Check sheet for the drawn part. Datum: minimum x, y, z corner. Units: mm. Round coordinates to 2 decimals unless told otherwise and drop trailing zeros. Write each loop counter-clockwise with the first axis right and the second up, starting at its lowest first coordinate (ties: lowest second). Pieces come first, ordered by that corner, then holes. Notation, with made-up numbers: (41, -27.75) - (98, -27.75) arc R27 ccw to (98, 5.25) - close; hole circle Ø6 at (81, 11). An arc over 180 degrees is marked (long way). Answer as a JSON object with one key per item and string values.
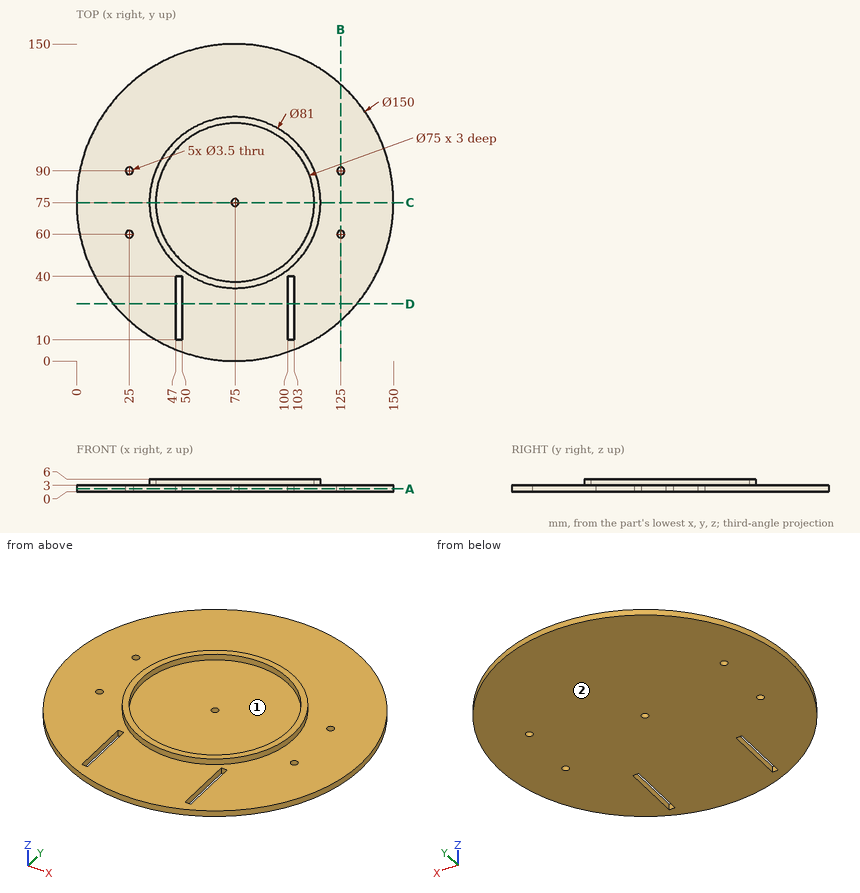
Q1. Section check A-A, the plane z = 1.35. Record the cut outline in (x, y), then the cut area to 3 significant figures.
Geometry check:
{"outline": "circle Ø150 at (75, 75); hole circle Ø3.5 at (25, 60); hole circle Ø3.5 at (25, 90); hole (47, 10) - (50, 10) - (50, 40) - (47, 40) - close; hole circle Ø3.5 at (75, 75); hole (100, 10) - (103, 10) - (103, 40) - (100, 40) - close; hole circle Ø3.5 at (125, 60); hole circle Ø3.5 at (125, 90)", "area": "17,400 mm2"}
Q2. Section check C-C, the plane y = 75. Record the cut outline in (x, z), then the cut area to 4 significant figures.
Geometry check:
{"outline": "(0, 0) - (73.25, 0) - (73.25, 3) - (37.5, 3) - (37.5, 6) - (34.5, 6) - (34.5, 3) - (0, 3) - close; (76.75, 0) - (150, 0) - (150, 3) - (115.5, 3) - (115.5, 6) - (112.5, 6) - (112.5, 3) - (76.75, 3) - close", "area": "457.5 mm2"}
Q3. Gauge pin test, flat ends, axial feed: P1, Ø3, axis at x = 25, y = 90, coming from the +Z side; P2, Ø0.9, axis at y = 24, z = 1, coming from the +X side; P3, Ø8, axis at x = 128.5, y = 95, coming from the +Z side; P4, Ø3.5, axis at y = 28.5, z = 1, coming from the -X side. Record the tip position at first contact, or that the pin passes through.
Geometry check:
{"P1": "passes through", "P2": "stops at x = 130.4", "P3": "stops at z = 3", "P4": "stops at x = 14.81"}
Q4. Section check D-D, the plane y = 27. Record the cut outline in (x, z).
Geometry check:
{"outline": "(17.37, 0) - (47, 0) - (47, 3) - (17.37, 3) - close; (50, 0) - (100, 0) - (100, 3) - (50, 3) - close; (103, 0) - (132.63, 0) - (132.63, 3) - (103, 3) - close"}
Q5. Release check for a two-part mould opening along X. For the marked faces 1 and 2 record: released by +X, released by -X, zero draft, split by the parting line, or undercut.
Geometry check:
{"face 1": "undercut", "face 2": "zero draft"}
Q6. Material ranges on line 1 along X through (y, z) = (90, 0.65); line 2 along Y through (x, z) = (25, 1.35); line 3 along X through (y, z) = (16, 1), recorded low to high. Write a range as [from, to].
Geometry check:
{"line 1": "x = [1.52, 23.25], [26.75, 123.25], [126.75, 148.48]", "line 2": "y = [19.1, 58.25], [61.75, 88.25], [91.75, 130.9]", "line 3": "x = [28.7, 47], [50, 100], [103, 121.3]"}
Q7. Section check B-B, the plane x = 125. Record the cut outline in (y, z).
Geometry check:
{"outline": "(19.1, 0) - (58.25, 0) - (58.25, 3) - (19.1, 3) - close; (61.75, 0) - (88.25, 0) - (88.25, 3) - (61.75, 3) - close; (91.75, 0) - (130.9, 0) - (130.9, 3) - (91.75, 3) - close"}
